Model file for the job. Use its own axes, mm. A direction names the side the tool comes from. Round coordinates to 2 decimals unless told otherwise and drop trailing zeros. Order: outer loops, then holes, each group sorted by start corner. A loop starts at its lowest first (then second) coordinate and runs counter-clockwise, first axis right, second up. Notation, with made-up numbers: (-39.75, 2.5) - (-8.75, 2.5) arc R17 cw to (-8.75, 27.5) - close; hole circle Ø4 at (45, 41.5). An arc over 180 degrees is marked (long way). Answer as CSV lines item,"result". Start each with the question number.
1. Pin check, flat tips, straight feed: pin 1 Ø1.7 at (x, z) = (0.5, 10) entering from +Y; pin 2 Ø2 at (y, z) = (-64, 8) entering from +X; pin 3 Ø8 at (x, z) = (-21.5, 5) entering from +Y (3 decimals). Stop position of each tip, or through.
2. Band-saw the part on A-A on x = 139. List the corners of the cut face in (y, z), then the cut area to 3 significant figures.
3. Band-saw the part on C-C on y = 117. List the corners of the cut face in (x, z), then the cut area to 3 significant figures.
4. Band-saw the part on B-B on y = -99.5. List the corners of the cut face in (x, z), then the cut area to 3 significant figures.
5. Band-saw the part on D-D on y = -40. List the corners of the cut face in (x, z), then the cut area to 3 significant figures.
6. Pull direction X, two halves, no side cores. Call faces 1 (the face through (-195.984, -53.67, 9.392)), 2 (the face through (127.83, 43.27, 9.39)), 3 (the face through (189.84, 65.97, 9.66)): released by +X, released by -X, zero draft, split by the parting line, or undercut.
7. 3-axis set-ups, long thin cutter, end or side, ignore diameter. For faces 4 (the face through (188.135, 46.662, 9.392)), 5 (the face through (80.655, -108.203, 9.392)), 6 (the face through (1.651, 131, 9)), 7 (the face through (-114.84, -164.78, 9.66)), 8 (the face through (121.23, -160.14, 9.66)): which of +Z, -Z, +X, -X, +Y, -Y reach the whole face in a straight line?
8. Wall check: line 1 along Y through (x, z) = (78.5, 3.5); line 2 along Y through (x, z) = (75.5, 5); line 3 along X through (y, z) = (-107.5, 16). Give the ranges that are in metal, low to high. Write a range as [from, to].
```python
from build123d import *

# Parameters (mm, degrees)
F1_DEPTH = 19.05
F3_DEPTH = 19.05
F4_R     = 7.62


# Not quite as in the source:
# - a length typed as a fraction of an inch, garbled in the dataset ("3 / 203.2 mm" for 3/8 in), is restored


with BuildPart() as f1:
    # F0 (on Top) → F1 (new body)
    with BuildSketch(Plane.XY):
        with BuildLine():
            Line((-72.9806935994, 21.976900663), (-193.7584921492, 61.2199862795))
            ThreePointArc((-193.7584921492, 61.2199862795), (-196.6172683272, -51.3019472882), (-139.1466642939, -148.0825641859))
            Line((-139.1466642939, -148.0825641859), (-109.9986790571, -148.5913441608))
            Line((-109.9986790571, -148.5913441608), (-46.1249232824, -60.6766615198))
            Line((-46.1249232824, -60.6766615198), (-43.453549167, -62.6175284229))
            Line((-43.453549167, -62.6175284229), (-118.0983337572, -165.3572603903))
            ThreePointArc((-118.0983337572, -165.3572603903), (-11.9670260336, -202.8473078153), (97.8362036413, -178.0963707015))
            Line((97.8362036413, -178.0963707015), (107.3273049417, -150.5322110638))
            Line((107.3273049417, -150.5322110638), (43.453549167, -62.6175284229))
            Line((43.453549167, -62.6175284229), (46.1249232824, -60.6766615198))
            Line((46.1249232824, -60.6766615198), (120.7697078726, -163.4163934872))
            ThreePointArc((120.7697078726, -163.4163934872), (189.2212394942, -74.064583468), (199.6127634745, 38.0129538194))
            Line((199.6127634745, 38.0129538194), (176.330601432, 55.5573213216))
            Line((176.330601432, 55.5573213216), (72.9806935994, 21.976900663))
            Line((72.9806935994, 21.976900663), (71.960319484, 25.1172892798))
            Line((71.960319484, 25.1172892798), (192.7381180338, 64.3603748963))
            ThreePointArc((192.7381180338, 64.3603748963), (128.9121834343, 157.0728778695), (25.5312687742, 201.5896681747))
            Line((25.5312687742, 201.5896681747), (1.651, 184.8685239645))
            Line((1.651, 184.8685239645), (1.651, 76.2))
            Line((1.651, 76.2), (-1.651, 76.2))
            Line((-1.651, 76.2), (-1.651, 203.1932927018))
            ThreePointArc((-1.651, 203.1932927018), (-109.5491285678, 171.1409607021), (-183.8335715961, 86.5763128934))
            Line((-183.8335715961, 86.5763128934), (-175.3102273166, 58.6977099385))
            Line((-175.3102273166, 58.6977099385), (-71.960319484, 25.1172892798))
            Line((-71.960319484, 25.1172892798), (-72.9806935994, 21.976900663))
        make_face()
    extrude(amount=F1_DEPTH)

    # F2 (on face) → F3 (cut, through all)
    with BuildSketch(Plane.XY.offset(19.05)):
        Polygon((3.6661742094, 6.35), (-3.6661742094, 6.35), (-7.3323484187, 0), (-3.6661742094, -6.35), (3.6661742094, -6.35), (7.3323484187, 0), align=None)
    extrude(amount=-F3_DEPTH, mode=Mode.SUBTRACT)

    # F4
    f4_edges = [f1.edges().sort_by_distance(p)[0] for p in [
        (-193.758492, 61.219986, 9.525),
        (-1.651, 203.193293, 9.525),
        (192.738118, 64.360375, 9.525),
        (120.769708, -163.416393, 9.525),
        (-118.098334, -165.35726, 9.525),
    ]]
    fillet(f4_edges, radius=F4_R)


solid = f1.part
```
Reply:
1,pin 1,"stops at y = 76.2"
1,pin 2,"stops at x = 193.19"
1,pin 3,"stops at y = 202.445"
2,outline,"(-148.22, 0) - (43.43, 0) - (43.43, 19.05) - (-148.22, 19.05) - close; (46.9, 0) - (148.22, 0) - (148.22, 19.05) - (46.9, 19.05) - close"
2,area,"5,580 mm2"
3,outline,"(-166.14, 0) - (-1.65, 0) - (-1.65, 19.05) - (-166.14, 19.05) - close; (1.65, 0) - (166.14, 0) - (166.14, 19.05) - (1.65, 19.05) - close"
3,area,"6,270 mm2"
4,outline,"(-177.17, 0) - (-74.33, 0) - (-74.33, 19.05) - (-177.17, 19.05) - close; (-70.25, 0) - (70.25, 0) - (70.25, 19.05) - (-70.25, 19.05) - close; (74.33, 0) - (177.17, 0) - (177.17, 19.05) - (74.33, 19.05) - close"
4,area,"6,590 mm2"
5,outline,"(-199.22, 0) - (199.22, 0) - (199.22, 19.05) - (-199.22, 19.05) - close"
5,area,"7,590 mm2"
6,face 1,"released by -X"
6,face 2,"undercut"
6,face 3,"released by +X"
7,face 4,"+Z, -Z, +X"
7,face 5,"+Z, -Z"
7,face 6,"+Z, -Z, +Y"
7,face 7,"+Z, -Z, -X"
7,face 8,"+Z, -Z, -Y"
8,line 1,"y = [-187.42, -110.85], [-105.24, 23.77], [27.24, 187.42]"
8,line 2,"y = [-188.65, -106.73], [-101.11, 22.8], [26.27, 188.65]"
8,line 3,"x = [-172.44, -80.14], [-76.06, 76.06], [80.14, 172.44]"
